Geometry check sheet. Reference: the model listing, model coordinates, mm. A direction names the side the tool comes from. Round coordinates to 2 decimals unless told otherwise and drop trailing zeros. Order: outer loops, then holes, each group sorted by start corner. A loop starts at its lowest first (then second) coordinate and runs counter-clockwise, first axis right, second up.
```python
from build123d import *

# Parameters (mm, degrees)
F2_W          = 300
F2_H          = 600
F3_DEPTH      = 30
F4_W          = 300
F4_H          = 600
F5_DEPTH      = 30
F6_W          = 30
F6_H          = 30
F7_DEPTH      = 860
F7_DEPTH_BACK = 860
F8_W          = 1780
F8_H          = 300
F9_DEPTH      = 1.5


with BuildPart() as f3:
    # F2 (on Right) → F3 (new body)
    with BuildSketch(Plane.YZ):
        with Locations((-150, 300)):
            Rectangle(F2_W, F2_H)
        Polygon((-270, 30), (-270, 281.45898), (-30, 401.45898), (-30, 30), align=None, mode=Mode.SUBTRACT)
        Polygon((-30, 570), (-30, 435), (-270, 315), (-270, 570), align=None, mode=Mode.SUBTRACT)
    extrude(amount=F3_DEPTH)



with BuildPart() as f5:
    # F4 (on offset) → F5 (new body)
    with BuildSketch(Plane.YZ.offset(1780)):
        with Locations((-150, 300)):
            Rectangle(F4_W, F4_H)
        Polygon((-270, 30), (-270, 281.45898), (-30, 401.45898), (-30, 30), align=None, mode=Mode.SUBTRACT)
        Polygon((-30, 570), (-30, 435), (-270, 315), (-270, 570), align=None, mode=Mode.SUBTRACT)
    extrude(amount=-F5_DEPTH)


with BuildPart() as f3_1:
    add(f3.part)

    add(f5.part)  # F7 merges F5
    # F6 (on offset) → F7 (join, two sides)
    with BuildSketch(Plane.YZ.offset(890)) as f7_sk:
        Polygon((-273.167184, 313.416408), (-300, 300), (-286.583592, 273.167184), (-259.750776, 286.583592), align=None)
        with Locations((-15, 585)):
            Rectangle(F6_W, F6_H)
        with Locations((-285, 585)):
            Rectangle(F6_W, F6_H)
        Polygon((-100.98995, 399.505025), (-127.822766, 386.088617), (-114.406358, 359.255801), (-87.573542, 372.672209), align=None)
    extrude(amount=F7_DEPTH)
    extrude(f7_sk.sketch, amount=-F7_DEPTH_BACK)

    # F8 (on face) → F9 (join)
    with BuildSketch(Plane.XY.offset(600)):
        with Locations((890, -150)):
            Rectangle(F8_W, F8_H)
    extrude(amount=F9_DEPTH)


solid = f3_1.part
```
(1) Sectioned sample at C-C, the plane y = -63. Record the cut outline in (x, z), and give its area (3 significant figures).
Returned:
outline: (0, 0) - (30, 0) - (30, 30) - (0, 30) - close; (0, 384.96) - (30, 384.96) - (30, 418.5) - (0, 418.5) - close; (0, 570) - (30, 570) - (30, 600) - (1750, 600) - (1750, 570) - (1780, 570) - (1780, 601.5) - (0, 601.5) - close; (1750, 0) - (1780, 0) - (1780, 30) - (1750, 30) - close; (1750, 384.96) - (1780, 384.96) - (1780, 418.5) - (1750, 418.5) - close
area: 8,280 mm2
(2) Sectioned sample at A-A, the plane x = 1533. Record the cut outline in (y, z).
Returned:
outline: (-300, 300) - (-286.58, 273.17) - (-259.75, 286.58) - (-273.17, 313.42) - close; (-300, 570) - (-270, 570) - (-270, 600) - (-30, 600) - (-30, 570) - (0, 570) - (0, 601.5) - (-300, 601.5) - close; (-127.82, 386.09) - (-114.41, 359.26) - (-87.57, 372.67) - (-100.99, 399.51) - close
(3) Sectioned sample at B-B, the plane z = 215.5. Record the cut outline in (x, y), and give its area (3 significant figures).
Returned:
outline: (0, -300) - (30, -300) - (30, -270) - (0, -270) - close; (0, -30) - (30, -30) - (30, 0) - (0, 0) - close; (1750, -300) - (1780, -300) - (1780, -270) - (1750, -270) - close; (1750, -30) - (1780, -30) - (1780, 0) - (1750, 0) - close
area: 3,600 mm2
(4) Depth check by flat-ended pin: P1, Ø6, axis at x = 1319, y = -162, coming from the -Z side; P2, Ø4, axis at x = 695.5, y = -89.5, coming from the -Z side; P3, Ø24, axis at x = 803, y = -15, coming from the -Z side. Enter the tip coordinate at first touch or a pass-through.
Returned:
P1: stops at z = 600
P2: stops at z = 370.71
P3: stops at z = 570
(5) Material ranges on line 1 (X direction, y = -25, z = 236); line 2 (Z direction, x = 930, y = -72); line 3 (Z direction, x = 832, y = -101.5), recorded low to high.
Returned:
line 1: x = 0 to 30, 1750 to 1780
line 2: z = 600 to 601.5
line 3: z = 365.71 to 399.25, 600 to 601.5
(6) Set-up check for faces 1 (the flat face through (878, -148, 600)), 2 (the flat face through (1765, -152, 0)), 3 (the flat face through (1765, -148, 30)): record each of +Z, -Z, +X, -X, +Y, -Y from which the full face is reachable in a straight line by a thin tool's end or side.
Returned:
face 1: none
face 2: -Z, +X, -X, +Y, -Y
face 3: +X, -X
(7) Draft check along Z on faces 4 (the flat face through (688.1, -122.8, 388.6)), 5 (the flat face through (15, -152, 0)), 6 (the flat face through (15, -270, 441)), 7 (the flat face through (878, -148, 601.5)). Enter one of: released by +Z, released by -Z, zero draft, split by the parting line, or undercut.
Returned:
face 4: undercut
face 5: released by -Z
face 6: undercut
face 7: released by +Z
